from build123d import *

# Parameters (mm, degrees)
F0_W     = 132.096782
F0_H     = 79.294358
F1_DEPTH = 25
F2_R     = 7.148366
F2_R_2   = 9.678364
F3_DEPTH = 25
F2_R_3   = 6.654601
F2_W     = 60.604844
F2_H     = 33.024194
F4_DEPTH = 25
F5_R     = 7.447322
F6_DEPTH = 25
F7_R     = 6.960859
F8_DEPTH = 25


with BuildPart() as f1:
    # F0 (on Top) → F1 (new body)
    with BuildSketch(Plane.XY):
        with Locations((-0.997983, -2.540322)):
            Rectangle(F0_W, F0_H)
    extrude(amount=F1_DEPTH)

    # F2 (on face) → F3 (cut)
    with BuildSketch(Plane.XY.offset(25)):
        with Locations((-55.614922, 27.852824)):
            Circle(F2_R)
        with Locations((-42.368952, -20.231856)):
            Circle(F2_R_2)
    extrude(amount=-F3_DEPTH, mode=Mode.SUBTRACT)

    # F2 (on face) → F4 (cut)
    with BuildSketch(Plane.XY.offset(25)):
        with Locations((-55.614922, 27.852824)):
            Circle(F2_R)
        with Locations((-42.368952, -20.231856)):
            Circle(F2_R_2)
        with Locations((41.098792, 26.582664)):
            Circle(F2_R_3)
        with Locations((20.413308, -12.97379)):
            Rectangle(F2_W, F2_H)
    extrude(amount=-F4_DEPTH, mode=Mode.SUBTRACT)

    # F5 (on face) → F6 (cut)
    with BuildSketch(Plane.XZ.offset(42.187501)):
        with Locations((22.263901, 11.891413)):
            Circle(F5_R)
    extrude(amount=-F6_DEPTH, mode=Mode.SUBTRACT)

    # F7 (on face) → F8 (cut)
    with BuildSketch(Plane(origin=(0, 37.106857, 0), x_dir=(-1, 0, 0), z_dir=(0, 1, 0))):
        with Locations((-8.310321, 15.035793)):
            Circle(F7_R)
    extrude(amount=-F8_DEPTH, mode=Mode.SUBTRACT)


solid = f1.part
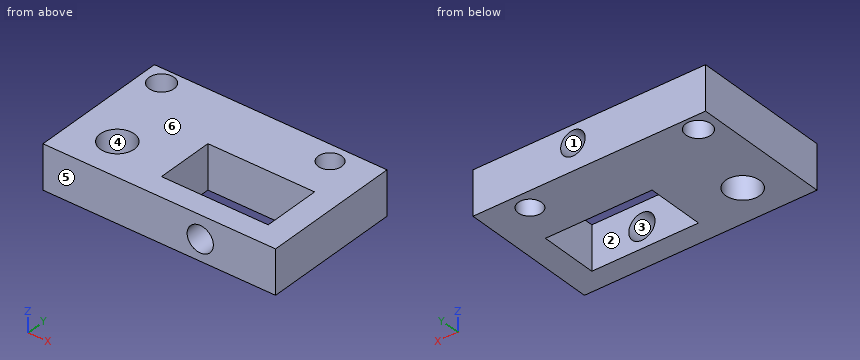
Model file for the job. Use its own axes, mm. Face numbers are marked on the shaded views. A direction names the side the tool comes from. Give positions to 0.01 mm unless a question says otherwise; leave off trailing zeros. Order: outer loops, then holes, each group sorted by start corner. A loop starts at its lowest first (then second) coordinate and runs counter-clockwise, first axis right, second up. Notation, with made-up numbers: M 68.25,11.25 L 118.25,11.25 A14 cw 118.25,17.25 Z; hole C -10,77 d1. An arc over 180 degrees is marked long. Put each result on its own line as item: value. Start each with the question number.
(1) Band-saw the part on B-B on y = -4.5. Give the cut face in (x, z).
(2) Pull direction Y, two halves, no side cores. Call the marked faces 4, 5 and 6: released by +Y, released by -Y, zero draft, split by the parting line, or undercut.
(3) Drill centre lines: L1, parallel to X at y = -21, z = 8.75; L2, parallel to Y at x = -5, z = 7.25; L3, parallel to X at y = -10, z = 13.25. Where is each one in solid material? Low to high. Write a range as [from, to].
(4) Tool access for the marked faces 1, 2 and 3: list every direction of +Z, -Z, +X, -X, +Y, -Y with a clear straight run to the whole face (end or side of a thin tool).
(5) Band-saw the part on A-A on x = -6. Give the cut face in (y, z).
(6) Band-saw the part on D-D on y = -18. Give the cut face in (x, z).
(7) Band-saw the part on C-C on z = 10. Give the cut face in (x, y).
(8) Pin check, flat tips, straight feed: pin 1 Ø13 at (x, y) = (-55.61, 27.85) entering from -Z; pin 2 Ø12 at (x, z) = (22.26, 11.89) entering from -Y. Stop position of each tip, or through.
Results below:
1. outline: M -67.05,0 L -9.89,0 L -9.89,25 L -67.05,25 Z; M 50.72,0 L 65.05,0 L 65.05,25 L 50.72,25 Z
2. face 4: undercut
2. face 5: released by -Y
2. face 6: zero draft
3. L1: x = [-67.05, -52.02], [-32.72, -9.89], [50.72, 65.05]
3. L2: y = [-42.19, -29.49], [3.54, 37.11]
3. L3: x = [-67.05, -9.89], [50.72, 65.05]
4. face 1: +Y
4. face 2: +Z, -Z
4. face 3: -Y
5. outline: M -42.19,0 L -29.49,0 L -29.49,25 L -42.19,25 Z; M 3.54,0 L 37.11,0 L 37.11,25 L 3.54,25 Z
6. outline: M -67.05,0 L -51.79,0 L -51.79,25 L -67.05,25 Z; M -32.95,0 L -9.89,0 L -9.89,25 L -32.95,25 Z; M 50.72,0 L 65.05,0 L 65.05,25 L 50.72,25 Z
7. outline: M -67.05,-42.19 L 15.06,-42.19 L 15.06,-29.49 L -9.89,-29.49 L -9.89,3.54 L 50.72,3.54 L 50.72,-29.49 L 29.47,-29.49 L 29.47,-42.19 L 65.05,-42.19 L 65.05,37.11 L 13.12,37.11 L 13.12,12.11 L 3.5,12.11 L 3.5,37.11 L -67.05,37.11 Z; hole C -55.61,27.85 d14.3; hole C -42.37,-20.23 d19.36; hole C 41.1,26.58 d13.31
8. pin 1: passes through
8. pin 2: stops at y = 3.54
